The model under review builds one solid part; all positions refer to its coordinate system, in mm. A direction names the side the tool comes from. Coordinates: 2 decimals unless noted, no trailing zeros. Loops run counter-clockwise (first coordinate to the right, second up) from the corner with the lowest first, then second, coordinate; pieces in that order, holes last. Notation, with made-up numbers: M 10.25,46 L 35.25,46 A20 cw 35.25,59 Z; hole C 61,-35.5 d11. An arc over 180 degrees is marked long. Return JSON: item names as keys, results as strings.
```python
from build123d import *

# Parameters (mm, degrees)
SKETCH1_R               = 31.5
SKETCH1_R_2             = 15.5
BOSS_EXTRUDE1_DEPTH     = 10
SKETCH1_3_R             = 15.5
BOSS_EXTRUDE2_DEPTH     = 4
SKETCH2_R               = 3.5
CUT_EXTRUDE1_DEPTH      = 47.695824224
SKETCH3_R               = 5
SKETCH3_R_2             = 3
CUT_EXTRUDE2_DEPTH      = 7
SKETCH3_4_R             = 3
CUT_EXTRUDE3_DEPTH      = 47.695824224
CUT_EXTRUDE3_DEPTH_BACK = 47.695824224


with BuildPart() as part:
    # Sketch1 → Boss-Extrude1 (new body)
    with BuildSketch(Plane.XY):
        Circle(SKETCH1_R)
        Circle(SKETCH1_R_2, mode=Mode.SUBTRACT)
        Circle(SKETCH1_R_2)
    extrude(amount=BOSS_EXTRUDE1_DEPTH)

    # Sketch1_3 → Boss-Extrude2 (add)
    with BuildSketch(Plane.XY):
        Circle(SKETCH1_3_R)
    extrude(amount=-BOSS_EXTRUDE2_DEPTH)

    # Sketch2 → Cut-Extrude1 (cut, through all)
    with BuildSketch(Plane(origin=(0, 0, -4), x_dir=(-1, 0, 0), z_dir=(0, 0, -1))):
        Circle(SKETCH2_R)
    extrude(amount=-CUT_EXTRUDE1_DEPTH, mode=Mode.SUBTRACT)

    # Sketch3 → Cut-Extrude2 (cut)
    with BuildSketch(Plane.XY.offset(10)):
        with Locations((-25, 0)):
            Circle(SKETCH3_R)
        with Locations((-25, 0)):
            Circle(SKETCH3_R_2, mode=Mode.SUBTRACT)
        with Locations(Location((25, 0, 0), (0, 0, 180))):
            Circle(SKETCH3_R)
        with Locations((0, 25)):
            Circle(SKETCH3_R)
        with Locations((0, 25)):
            Circle(SKETCH3_R_2, mode=Mode.SUBTRACT)
        with Locations((0, -25)):
            Circle(SKETCH3_R)
        with Locations((0, -25)):
            Circle(SKETCH3_R_2, mode=Mode.SUBTRACT)
    extrude(amount=-CUT_EXTRUDE2_DEPTH, mode=Mode.SUBTRACT)

    # Sketch3_4 → Cut-Extrude3 (cut, two sides)
    with BuildSketch(Plane.XY.offset(10)) as cut_extrude3_sk:
        with Locations((-25, 0)):
            Circle(SKETCH3_4_R)
        with Locations((25, 0)):
            Circle(SKETCH3_4_R)
        with Locations((0, 25)):
            Circle(SKETCH3_4_R)
        with Locations((0, -25)):
            Circle(SKETCH3_4_R)
    extrude(amount=CUT_EXTRUDE3_DEPTH, mode=Mode.SUBTRACT)
    extrude(cut_extrude3_sk.sketch, amount=-CUT_EXTRUDE3_DEPTH_BACK, mode=Mode.SUBTRACT)


solid = part.part
```
1. To check wall thickness, follow line 1 (Y direction, x = 0, z = 1.1); line 2 (Y direction, x = 2, z = 3.25); line 3 (Z direction, x = 19, y = -25). State the ranges of each line that lie inside material, in increasing order.
Check values:
{"line 1": "-31.5 to -28, -22 to -3.5, 3.5 to 22, 28 to 31.5", "line 2": "-31.44 to -29.58, -20.42 to -2.87, 2.87 to 20.42, 29.58 to 31.44", "line 3": "0 to 10"}
2. Add section D-D on x = 26. Give the boundary of the cut face in (y, z), plus the area to 3 significant figures.
Check values:
{"outline": "M -17.78,0 L -2.83,0 L -2.83,3 L -4.9,3 L -4.9,10 L -17.78,10 Z; M 2.83,0 L 17.78,0 L 17.78,10 L 4.9,10 L 4.9,3 L 2.83,3 Z", "area": "270 mm²"}
3. The part is to be moulded in two halves that separate along X. For faces 4 (the face through (7, 14, 0)), 5 (the face through (-25.1, -3.3, 3)), 6 (the face through (-1.08, 20.12, 6.55)), 7 (the face through (-4.101, 31.232, 4.93)), say which applies: released by +X, released by -X, zero draft, split by the parting line, or undercut.
Check values:
{"face 4": "zero draft", "face 5": "undercut", "face 6": "undercut", "face 7": "split by the parting line"}
4. Add section A-A on x = 0. Give the boundary of the cut face in (y, z).
Check values:
{"outline": "M -31.5,0 L -28,0 L -28,3 L -30,3 L -30,10 L -31.5,10 Z; M -22,0 L -15.5,0 L -15.5,-4 L -3.5,-4 L -3.5,10 L -20,10 L -20,3 L -22,3 Z; M 3.5,-4 L 15.5,-4 L 15.5,0 L 22,0 L 22,3 L 20,3 L 20,10 L 3.5,10 Z; M 28,0 L 31.5,0 L 31.5,10 L 30,10 L 30,3 L 28,3 Z"}
5. Insertion check: pin 1 Ø1 at (x, z) = (-14.5, 3.5) entering from -Y; pin 2 Ø8 at (x, z) = (-11.5, -0.5) entering from -Y; pin 3 Ø1.5 at (x, y) = (7, 17.5) entering from -Z; pin 4 Ø3.5 at (x, y) = (25, 0) entering from -Z. Each pin has a flat end and moves straight along its axis. Give the tip position at first contact, or say it passes through.
Check values:
{"pin 1": "y = -28.22", "pin 2": "y = -30.59", "pin 3": "z = 0", "pin 4": "through"}
6. Machinability: for faces 1 (the face through (-0.1, -28.3, 3)), 2 (the face through (7, 0, 10)), 3 (the face through (-2.018, 15.368, -1.972)), which of the approach directions +Z, -Z, +X, -X, +Y, -Y give a long, thin tool a straight path to every point of the face, cutting with its end or side? Answer none if there is none.
Check values:
{"face 1": "+Z", "face 2": "+Z, +X, -X, +Y, -Y", "face 3": "-Z"}
7. Add section C-C on z = 4.5. Give the boundary of the cut face in (x, y), plus the area to 3 significant figures.
Check values:
{"outline": "C 0,0 d63; hole C -25,0 d10; hole C 0,-25 d10; hole C 0,25 d10; hole C 0,0 d7; hole C 25,0 d10", "area": "2,760 mm²"}
